Solid Edge part; units mm, degrees
sketch "Sketch1" plane through (0, 0, 0) normal (0, 0, 1) x (1, 0, 0)
  line L0 (66.4689, 35.8597) -> (-66.4689, 35.8597)
  line L1 (-66.4689, 35.8597) -> (-66.4689, -35.8597)
  line L2 (-66.4689, -35.8597) -> (66.4689, -35.8597)
  line L3 (66.4689, -35.8597) -> (66.4689, 35.8597)
extrude "Protrusion1" add sketch "Sketch1" along normal blind 90
hole "Hole_1" at (-44.8515, -15.5036, 90) direction (0, 0, -1) diameter 10 end up to next
hole "Hole1" at (44.8515, -15.5036, 90) direction (0, 0, -1) diameter 10 end up to next
hole "Hole2" at (44.8515, 15.5036, 90) direction (0, 0, -1) diameter 10 end up to next
hole "Hole3" at (-44.8515, 15.5036, 90) direction (0, 0, -1) diameter 10 end up to next
Check sheet for the modelled part. Datum: model origin and axes. Units: mm. Give positions to 0.01 mm unless a question says otherwise; leave off trailing zeros. Write each loop counter-clockwise with the first axis right and the second up, starting at its lowest first coordinate (ties: lowest second). Pieces come first, ordered by that corner, then holes. Notation, with made-up numbers: (40, 29) -> (46, 29) arc R13 cw to (46, 37) -> close; hole circle Ø1 at (-28, 73). An arc over 180 degrees is marked (long way). Use one line per item in the form item = value. Start each with the question number.
1. Mould release check, pull along Y, two halves, no side actions. Record for faces 1 (the cylindrical face through (-47.894, 19.471, 45.63)), 2 (the flat face through (66.469, -1, 44)), 3 (the flat face through (-1, -35.86, 44)): pulls with the +Y half, pulls with the -Y half, needs draft (parallel to the pull), parting line crosses it, or undercut.
2. Thickness scan on line 1 along Y through (x, z) = (45, 29.5); line 2 along Y through (x, z) = (42.5, 79); line 3 along X through (y, z) = (17, 40.5). Record the ranges inside material, lowest first. Write a range as from..to.
3. Section check A-A (y = 18). Record the cut outline in (x, z), and give its area (3 significant figures).
4. Go/stop test with a flat-tipped pin: P1, Ø16, axis at x = -44.85, y = 15.5, coming from the -Z side. Record where the tip stops, or that it passes through.
5. Section check B-B (z = 63.5). Record the cut outline in (x, y), and give its area (3 significant figures).
Conclusion:
q1.face_1 = undercut
q1.face_2 = needs draft
q1.face_3 = pulls with the -Y half
q2.line_1 = -35.86..-20.5, -10.51..10.51, 20.5..35.86
q2.line_2 = -35.86..-19.92, -11.09..11.09, 19.92..35.86
q2.line_3 = -66.47..-49.62, -40.08..40.08, 49.62..66.47
q3.outline = (-66.47, 0) -> (-49.18, 0) -> (-49.18, 90) -> (-66.47, 90) -> close; (-40.52, 0) -> (40.52, 0) -> (40.52, 90) -> (-40.52, 90) -> close; (49.18, 0) -> (66.47, 0) -> (66.47, 90) -> (49.18, 90) -> close
q3.area = 10,400 mm²
q4.P1 = 0
q5.outline = (-66.47, -35.86) -> (66.47, -35.86) -> (66.47, 35.86) -> (-66.47, 35.86) -> close; hole circle Ø10 at (-44.85, -15.5); hole circle Ø10 at (-44.85, 15.5); hole circle Ø10 at (44.85, -15.5); hole circle Ø10 at (44.85, 15.5)
q5.area = 9,220 mm²
